```python
from build123d import *

# Parameters (mm, degrees)
F0_R     = 5.9817
F1_DEPTH = 25.4
F2_R     = 5.207
F3_DEPTH = 12.7
F4_SIZE2 = 1.8330871047
F4_SIZE  = 3.175
F5_SIZE2 = 0.4399409051
F5_SIZE  = 0.762
F7_D     = 5.1054
F7_DEPTH = 19.05
F7_TIP   = 1.5338169022


with BuildPart() as f1:
    # F0 (on Top) → F1 (new body, symmetric)
    with BuildSketch(Plane.XY):
        Circle(F0_R)
    extrude(amount=F1_DEPTH, both=True)

    # F2 (on face) → F3 (join)
    with BuildSketch(Plane.XY.offset(25.4)):
        Circle(F2_R)
    extrude(amount=F3_DEPTH)

    # F4
    f4_edges = [f1.edges().sort_by_distance(p)[0] for p in [
        (-5.207, 0, 38.1),
    ]]
    f4_side = f1.faces().sort_by_distance((-5.207, 0, 31.75))[0]
    chamfer(f4_edges, length=F4_SIZE, length2=F4_SIZE2, reference=f4_side)

    # F5
    f5_edges = [f1.edges().sort_by_distance(p)[0] for p in [
        (-5.9817, 0, -25.4),
    ]]
    f5_side = f1.faces().sort_by_distance((-5.9817, 0, 0))[0]
    chamfer(f5_edges, length=F5_SIZE, length2=F5_SIZE2, reference=f5_side)

    # F7
    with Locations(Plane(origin=(0, 0, -25.4), x_dir=(1, 0, 0), z_dir=(0, 0, -1))):
        with Locations((0, 0)):
            Hole(F7_D / 2, depth=F7_DEPTH)
            with Locations((0, 0, -(F7_DEPTH + F7_TIP / 2))):  # 118° drill point
                Cone(0, F7_D / 2, F7_TIP, mode=Mode.SUBTRACT)


solid = f1.part
```
The listing builds one solid part. Answer for the finished solid, in the listing's coordinates (mm). Coordinates: 2 decimals unless noted, no trailing zeros. Write each loop counter-clockwise with the first axis right and the second up, starting at its lowest first coordinate (ties: lowest second). Pieces come first, ordered by that corner, then holes. Notation, with made-up numbers: M 21.5,-7.5 L 31.5,-7.5 A3 ccw 31.5,-2.5 Z; hole C 71,11 d9. An arc over 180 degrees is marked long. Use a Markdown table: item, result. Add a question column.
1. Section A-A (z = 20) is taken. Give the vertices of the cut face in (x, y).
2. For a pull along Y with two mould halves and no side action, classify faces 1 (the cylindrical face through (4.967, 1.564, 30.096)), 2 (the flat face through (-2, 5, 25.4)), 3 (the cylindrical face through (-2.435, -0.767, -15.742)) as +Y half, -Y half, draft (parallel to the pull), parting line (faces both ways), or undercut.
3. Given P1, Ø3, axis at y = 2, z = 0.5, coming from the -X side; P2, Ø1.5, axis at x = 4.5, z = 30.5, coming from the -Y side; P3, Ø1.5, axis at x = 2, y = -4, coming from the +Z side, each flat-ended and moving along its own axis, determine where each tip first touches the part or whether it passes through.
4. Straight lines are drawn through the part: line 1 along Y through (x, z) = (0, -11); line 2 along X through (y, z) = (-1.5, -11); line 3 along Z through (x, y) = (2.25, 4.75). For each, find the intervals that lie inside material, in ascending order. Write a range as [from, to].
Data:
| question | item | result |
|---|---|---|
| 1 | outline | C 0,0 d11.96 |
| 2 | face 1 | parting line |
| 2 | face 2 | draft |
| 2 | face 3 | undercut |
| 3 | P1 | stops at x = -5.96 |
| 3 | P2 | stops at y = -3.61 |
| 3 | P3 | stops at z = 37.5 |
| 4 | line 1 | y = [-5.98, -2.55], [2.55, 5.98] |
| 4 | line 2 | x = [-5.79, -2.07], [2.07, 5.79] |
| 4 | line 3 | z = [-25.4, 25.4] |
